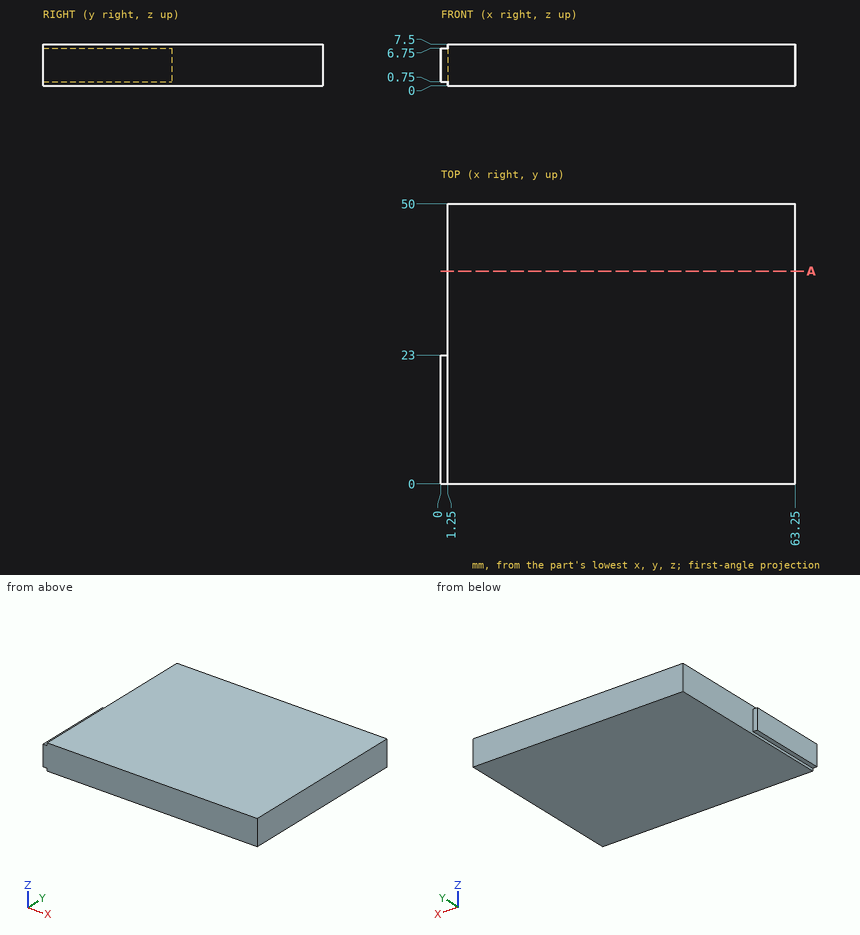
Can you work these out from the drawing? Everything is in mm from the part's minimum corner. Give positions to 0.01 mm unless a question says otherwise; leave off trailing zeros. Order: outer loops, then holes, each group sorted by start corner. A loop starts at its lowest first (then second) coordinate and runs counter-clockwise, first axis right, second up.
Item 1: I need wall thicknesses on line 1 (X direction, y = 42, z = 2). Which ranges of the line are inside material? Lowest first, please.
Item 2: If we section it at A-A, the plane y = 38: Write out the boundary of the cut face in (x, z).
Item 3: I'm going to push flat-ended pins straight in: pin 1 (1 mm diameter, centred on x = 0.5, z = 3, fed in from +Y); pin 2 (2 mm diameter, centred on y = 28.5, z = 6, fed in from -X); pin 3 (1.4 mm diameter, centred on x = 0.5, y = 8.5, fed in from -Z). Where does each tip first touch, or does it pass through?
Values:
1. line 1: x = 1.25 to 63.25
2. outline: (1.25, 0) - (63.25, 0) - (63.25, 7.5) - (1.25, 7.5) - close
3. pin 1: stops at y = 23
3. pin 2: stops at x = 1.25
3. pin 3: stops at z = 0.75
